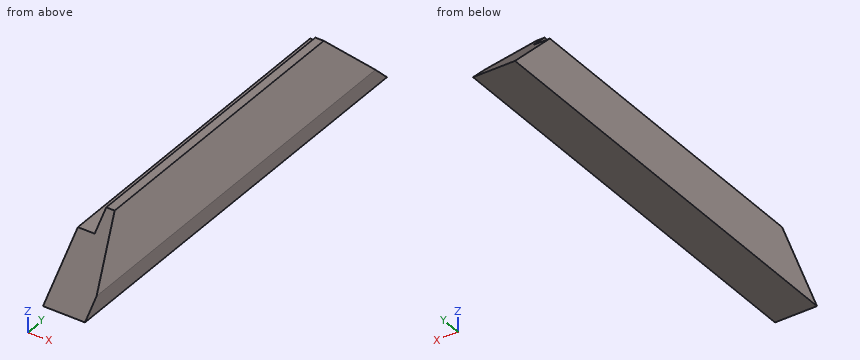
```python
from build123d import *

# Parameters (mm, degrees)
F0_W     = 165.1
F0_H     = 25.4
F1_DEPTH = 15.875
F3_W     = 6.35
F3_H     = 6.35
F4_DEPTH = 165.101
F5_DEPTH = 15.876
F6_SIZE2 = 6.348172
F6_SIZE  = 19.05


with BuildPart() as f1:
    # F0 (on Right) → F1 (new body)
    with BuildSketch(Plane.YZ):
        with Locations((2.164774, 0)):
            Rectangle(F0_W, F0_H)
    extrude(amount=F1_DEPTH)

    # F3 (on face) → F4 (cut, through all)
    with BuildSketch(Plane.XZ.offset(80.385226)):
        with Locations((3.175, 9.525)):
            Rectangle(F3_W, F3_H)
    extrude(amount=-F4_DEPTH, mode=Mode.SUBTRACT)

    # F2 (on face) → F5 (cut, through all)
    with BuildSketch(Plane.YZ.offset(15.875)):
        Polygon((-80.385226, 12.7), (-80.385226, -12.7), (-54.985226, 12.7), align=None)
        Polygon((59.314774, 12.7), (84.714774, -12.7), (84.714774, 12.7), align=None)
    extrude(amount=-F5_DEPTH, mode=Mode.SUBTRACT)

    # F6
    f6_edges = [f1.edges().sort_by_distance(p)[0] for p in [
        (15.875, 2.164774, 12.7),
    ]]
    chamfer(f6_edges, length=F6_SIZE, length2=F6_SIZE2)


solid = f1.part
```
For this review, take the finished solid that the model builds, in its own axes (mm). Give positions to 0.01 mm unless a question says otherwise; leave off trailing zeros. Write each loop counter-clockwise with the first axis right and the second up, starting at its lowest first coordinate (ties: lowest second). Pieces come first, ordered by that corner, then holes.
Item 1: Insertion check: P1, Ø1.9, axis at x = 4, y = 1.5, coming from the +Z side; P2, Ø2, axis at y = -15, z = -4.5, coming from the -X side; P3, Ø1, axis at x = 7, z = -9, coming from the -Y side; P4, Ø4, axis at x = 13.5, z = 6.5, coming from the -Y side. Each pin has a flat end and moves straight along its axis. Give the tip position at first contact, or say it passes through.
Item 2: Take a section at A-A (y = -16.5). Give the boundary of the cut face in (x, z) (3 decimals).
Item 3: Take a section at D-D (y = -57). Give the boundary of the cut face in (x, z) (3 decimals).
Item 4: Take a section at C-C (z = -9.25). Give the boundary of the cut face in (x, y) (3 decimals).
Item 5: Take a section at B-B (x = 1.5). Give the boundary of the cut face in (y, z), and give its area (3 significant figures).
Item 6: Wall thickness on probe 1 along Z at (x, y) = (2, -29); probe 2 along Y at (x, z) = (12.75, -10); probe 3 along Y at (x, z) = (8, 8.5): over which ranges is each line inside the solid? List them lowest first.
Established:
1. P1: stops at z = 6.35
1. P2: stops at x = 0
1. P3: stops at y = -77.19
1. P4: stops at y = -62.57
2. outline: (0, -12.7) - (15.875, -12.7) - (15.875, -6.35) - (9.527, 12.7) - (6.35, 12.7) - (6.35, 6.35) - (0, 6.35) - close
3. outline: (0, -12.7) - (15.875, -12.7) - (15.875, -6.35) - (10.198, 10.685) - (6.35, 10.685) - (6.35, 6.35) - (0, 6.35) - close
4. outline: (0, -76.935) - (15.875, -76.935) - (15.875, 81.265) - (0, 81.265) - close
5. outline: (-80.39, -12.7) - (84.71, -12.7) - (65.66, 6.35) - (-61.34, 6.35) - close
5. area: 2,780 mm2
6. probe 1: z = -12.7 to 6.35
6. probe 2: y = -77.69 to 82.01
6. probe 3: y = -59.19 to 63.51
